Geometry check sheet. Reference: the model listing, model coordinates, mm. A direction names the side the tool comes from. Round coordinates to 2 decimals unless told otherwise and drop trailing zeros. Order: outer loops, then holes, each group sorted by start corner. A loop starts at its lowest first (then second) coordinate and runs counter-clockwise, first axis right, second up.
(1) Cross-section at D-D on z = 228. Enter the section's corners in (x, y).
(2) Draft check along X on faces 4 (the face through (-604, -72, 163.527)), 5 (the face through (-241.3, -53, -2)), 6 (the face through (-254.48, 11.67, -149.72)). Enter one of: pulls with the +X half, pulls with the -X half, needs draft (parallel to the pull), parting line crosses it, or undercut.
(3) Gauge pin test, flat ends, axial feed: P1, Ø3.5, axis at x = -476.5, y = -41.5, coming from the -Z side; P2, Ø6.5, axis at x = -483.5, z = -130.5, coming from the +Y side; P3, Ø10, axis at x = -295, y = -9, coming from the -Z side; P4, Ø8, axis at x = -544.5, y = -20, coming from the -Z side. Record the tip position at first contact, or that the pin passes through.
(4) Cross-section at A-A on z = -188. Enter the section's corners in (x, y).
(5) Set-up check for faces 1 (the face through (-484, -69, -180.167)), 2 (the face through (-479.22, -93.84, 321.89)), 3 (the face through (-268.033, -19, -65)): record each of +Z, -Z, +X, -X, +Y, -Y from which the full face is reachable in a straight line by a thin tool's end or side.
(6) Cross-section at C-C on z = 12. Enter the section's corners in (x, y), and give its area (3 significant figures).
(7) Cross-section at B-B on x = -434.5. Enter the section's corners in (y, z), and give its area (3 significant figures).
(8) Thickness scan on L1, parallel to X at y = -48, z = -195.5; L2, parallel to X at y = -18.5, z = -212; L3, parallel to Z at x = -584, y = -63. Record the ranges inside material, lowest first.
from build123d import *

# Parameters (mm, degrees)
F1_DEPTH  = 120.65
F2_R      = 9.9885996102
F2_R_2    = 10.5258660688
F3_DEPTH  = 482.6
F4_W      = 344.8911011219
F4_H      = 764.6993398666
F4_W_2    = 120.65
F4_H_2    = 673.1
F5_DEPTH  = 482.6
F8_W      = 431.8
F8_H      = 584.2
F9_DEPTH  = 50.8
F10_W     = 19.05
F10_H     = 19.05
F11_DEPTH = 95.25
F10_W_2   = 47.625
F10_H_2   = 22.225
F12_DEPTH = 3.175


with BuildPart() as f1:
    # F0 (on Front) → F1 (new body)
    with BuildSketch(Plane.XZ):
        with BuildLine():
            Line((-241.3, 323.85), (-241.3, -349.25))
            Line((-241.3, -349.25), (241.3, -349.25))
            Line((241.3, -349.25), (241.3, 323.85))
            ThreePointArc((241.3, 323.85), (0, 349.25), (-241.3, 323.85))
        make_face()
    extrude(amount=F1_DEPTH)

    # F4 (on face) → F5 (cut)
    with BuildSketch(Plane.YZ.offset(241.3)):
        with Locations((-53.2562285662, 11.3563537598)):
            Rectangle(F4_W, F4_H)
        with Locations((-60.325, -12.7)):
            Rectangle(F4_W_2, F4_H_2, mode=Mode.SUBTRACT)
        with Locations((-60.325, -12.7)):
            Rectangle(F4_W_2, F4_H_2)
    extrude(amount=-F5_DEPTH, mode=Mode.SUBTRACT)


with BuildPart() as f3:
    # F2 (on face) → F3 (new body)
    with BuildSketch(Plane(origin=(-241.3, 0, 0), x_dir=(0, -1, 0), z_dir=(-1, 0, 0))):
        with BuildLine():
            Line((0, -68.1404843926), (0, -233.649328351))
            ThreePointArc((0, -233.649328351), (21.350852379, -281.1488587038), (55.2847087383, -320.6527531147))
            ThreePointArc((55.2847087383, -320.6527531147), (84.0658754315, -337.5428209275), (115.3160259128, -349.25))
            ThreePointArc((115.3160259128, -349.25), (119.6951401667, -326.4048751593), (115.3160259128, -303.5597503185))
            ThreePointArc((115.3160259128, -303.5597503185), (101.3495716057, -189.7295194826), (93.6318859458, -75.3056555986))
            ThreePointArc((93.6318859458, -75.3056555986), (95.2968862194, 29.9638674769), (103.9162650704, 134.8931342363))
            ThreePointArc((103.9162650704, 134.8931342363), (108.0016932489, 216.2111774087), (103.9162650704, 297.5292205811))
            ThreePointArc((103.9162650704, 297.5292205811), (100.4192959768, 311.8158756468), (91.9625142686, 323.85))
            Line((91.9625142686, 323.85), (31.436908019, 323.85))
            ThreePointArc((31.436908019, 323.85), (31.1849940922, 323.6171736523), (30.9348870069, 323.3824074268))
            ThreePointArc((30.9348870069, 323.3824074268), (15.2328502157, 295.0276660156), (11.4129362628, 262.8414332867))
            ThreePointArc((11.4129362628, 262.8414332867), (15.6896829727, 217.6965972865), (24.1801738739, 173.1515824795))
            ThreePointArc((24.1801738739, 173.1515824795), (29.6284254011, 138.4055637112), (29.6032354236, 103.2349988818))
            ThreePointArc((29.6032354236, 103.2349988818), (16.9934129505, 17.1686486524), (0, -68.1404843926))
        make_face()
        with Locations((71.3824555278, -287.1399223804)):
            Circle(F2_R, mode=Mode.SUBTRACT)
        with Locations((60.1097382605, -151.0620862246)):
            Circle(F2_R_2, mode=Mode.SUBTRACT)
        with BuildLine():
            ThreePointArc((69.983959198, 334.6931636333), (49.4182050819, 333.8654070908), (31.436908019, 323.85))
            Line((31.436908019, 323.85), (91.9625142686, 323.85))
            ThreePointArc((91.9625142686, 323.85), (81.8305714463, 331.0093567724), (69.983959198, 334.6931636333))
        make_face()
        with BuildLine():
            ThreePointArc((0, -68.1404843926), (-11.673043687, -150.8949063718), (0, -233.649328351))
            Line((0, -233.649328351), (0, -68.1404843926))
        make_face()
    extrude(amount=F3_DEPTH)

    # F8 (on plane+point) → F9 (cut)
    with BuildSketch(Plane.XZ.offset(-11.673043687)):
        with Locations((-483.9325845242, 4.38026824)):
            Rectangle(F8_W, F8_H)
    extrude(amount=F9_DEPTH, mode=Mode.SUBTRACT)

    # F10 (on face) → F11 (cut)
    with BuildSketch(Plane(origin=(0, -39.126956313, 0), x_dir=(-1, 0, 0), z_dir=(0, 1, 0))):
        with Locations((364.0763345242, 173.05214324)):
            Rectangle(F10_W, F10_H)
        with Locations((483.9325845242, 173.05214324)):
            Rectangle(F10_W, F10_H)
        with Locations((603.7888345242, 173.05214324)):
            Rectangle(F10_W, F10_H)
        with Locations((364.0763345242, 50.02089324)):
            Rectangle(F10_W, F10_H)
        with Locations((483.9325845242, 50.02089324)):
            Rectangle(F10_W, F10_H)
        with Locations((603.7888345242, 50.02089324)):
            Rectangle(F10_W, F10_H)
        with Locations((603.7888345242, -66.66035676)):
            Rectangle(F10_W, F10_H)
        with Locations((483.9325845242, -66.66035676)):
            Rectangle(F10_W, F10_H)
        with Locations((364.0763345242, -66.66035676)):
            Rectangle(F10_W, F10_H)
        with Locations((364.0763345242, -189.69160676)):
            Rectangle(F10_W, F10_H)
        with Locations((483.9325845242, -189.69160676)):
            Rectangle(F10_W, F10_H)
        with Locations((603.7888345242, -189.69160676)):
            Rectangle(F10_W, F10_H)
    extrude(amount=-F11_DEPTH, mode=Mode.SUBTRACT)

    # F10 (on face) → F12 (cut)
    with BuildSketch(Plane(origin=(0, -39.126956313, 0), x_dir=(-1, 0, 0), z_dir=(0, 1, 0))):
        with Locations((364.0763345242, 111.53651824)):
            Rectangle(F10_W_2, F10_H_2)
        with Locations((483.9325845242, 111.53651824)):
            Rectangle(F10_W_2, F10_H_2)
        with Locations((603.7888345242, 111.53651824)):
            Rectangle(F10_W_2, F10_H_2)
        with Locations((364.0763345242, -8.31973176)):
            Rectangle(F10_W_2, F10_H_2)
        with Locations((483.9325845242, -8.31973176)):
            Rectangle(F10_W_2, F10_H_2)
        with Locations((603.7888345242, -8.31973176)):
            Rectangle(F10_W_2, F10_H_2)
        with Locations((603.7888345242, -128.17598176)):
            Rectangle(F10_W_2, F10_H_2)
        with Locations((483.9325845242, -128.17598176)):
            Rectangle(F10_W_2, F10_H_2)
        with Locations((364.0763345242, -128.17598176)):
            Rectangle(F10_W_2, F10_H_2)
    extrude(amount=-F12_DEPTH, mode=Mode.SUBTRACT)


solid = f3.part
Found:
1. outline: (-723.9, -107.92) - (-241.3, -107.92) - (-241.3, -14.34) - (-268.03, -14.34) - (-268.03, -39.13) - (-699.83, -39.13) - (-699.83, -14.34) - (-723.9, -14.34) - close
2. face 4: undercut
2. face 5: pulls with the +X half
2. face 6: needs draft
3. P1: stops at z = -309.14
3. P2: stops at y = -42.3
3. P3: passes through
3. P4: stops at z = 296.48
4. outline: (-723.9, -101.19) - (-613.31, -101.19) - (-613.31, -39.13) - (-699.83, -39.13) - (-699.83, 9.36) - (-723.9, 9.36) - close; (-594.26, -101.19) - (-493.46, -101.19) - (-493.46, -39.13) - (-594.26, -39.13) - close; (-474.41, -101.19) - (-373.6, -101.19) - (-373.6, -39.13) - (-474.41, -39.13) - close; (-354.55, -101.19) - (-241.3, -101.19) - (-241.3, 9.36) - (-268.03, 9.36) - (-268.03, -39.13) - (-354.55, -39.13) - close
5. face 1: +Y, -Y
5. face 2: +Z, +X, -X, -Y
5. face 3: +Y
6. outline: (-723.9, -94.52) - (-241.3, -94.52) - (-241.3, -16.09) - (-268.03, -16.09) - (-268.03, -39.13) - (-699.83, -39.13) - (-699.83, -16.09) - (-723.9, -16.09) - close
6. area: 27,900 mm2
7. outline: (-115.32, -349.25) arc R193.98 ccw to (-55.28, -320.65) arc R181.91 ccw to (-25.73, -287.72) - (-39.13, -287.72) - (-39.13, 296.48) - (-15.72, 296.48) arc R84.15 ccw to (-30.93, 323.38) arc R44.39 ccw to (-31.44, 323.85) arc R44.39 ccw to (-69.98, 334.69) arc R39.71 ccw to (-103.92, 297.53) arc R811.34 ccw to (-103.92, 134.89) arc R1591.98 cw to (-93.63, -75.31) arc R2095.36 cw to (-115.32, -303.56) arc R61.78 ccw to start; hole circle Ø19.98 at (-71.38, -287.14); hole circle Ø21.05 at (-60.11, -151.06)
7. area: 41,800 mm2
8. L1: x = -723.9 to -613.31, -594.26 to -493.46, -474.41 to -373.6, -354.55 to -241.3
8. L2: x = -723.9 to -699.83, -268.03 to -241.3
8. L3: z = -325.85 to -292.57, -281.71 to -161.18, -140.94 to 335.5
